from build123d import *

# Parameters (mm, degrees)
SKETCH1_W                                        = 76.2
SKETCH1_H                                        = 50.8
BOSS_EXTRUDE1_DEPTH                              = 11.79269038
BOSS_EXTRUDE2_START                              = -38.1
BOSS_EXTRUDE2_DEPTH                              = 19.05
F_1_4_CLEARANCE_HOLE2_D                          = 6.7564
CBORE_FOR_1_4_SOCKET_HEAD_CAP_SCREW1_D           = 6.7564
CBORE_FOR_1_4_SOCKET_HEAD_CAP_SCREW1_CBORE_D     = 11.1125
CBORE_FOR_1_4_SOCKET_HEAD_CAP_SCREW1_CBORE_DEPTH = 6.35


with BuildPart() as part:
    # Sketch1 → Boss-Extrude1 (new body)
    with BuildSketch(Plane(origin=(0, 0, 0), x_dir=(0, 0, -1), z_dir=(1, 0, 0))):
        Rectangle(SKETCH1_W, SKETCH1_H)
    extrude(amount=BOSS_EXTRUDE1_DEPTH)

    # Sketch7 → Boss-Extrude2 (add, symmetric)
    with BuildSketch(Plane.XY.offset(38.1).offset(BOSS_EXTRUDE2_START)):
        Polygon((11.79269038, -25.4), (49.89269038, -25.4), (49.89269038, 9.525), (43.54269038, 9.525), (43.54269038, -15.875), (11.79269038, -15.875), align=None)
    extrude(amount=BOSS_EXTRUDE2_DEPTH, both=True)

    # 1/4 Clearance Hole2 (through all)
    with Locations(Plane(origin=(49.89269038, 0, 0), x_dir=(0, 0, -1), z_dir=(1, 0, 0))):
        with Locations((-9.525, 3.175), (9.525, 3.175)):
            Hole(F_1_4_CLEARANCE_HOLE2_D / 2)

    # CBORE for 1/4 Socket Head Cap Screw1 (through all)
    with Locations(Plane(origin=(11.79269038, 0, 0), x_dir=(0, 0, -1), z_dir=(1, 0, 0))):
        with Locations((-28.575, 15.875), (28.575, 15.875), (28.575, -15.875), (-28.575, -15.875)):
            CounterBoreHole(CBORE_FOR_1_4_SOCKET_HEAD_CAP_SCREW1_D / 2, CBORE_FOR_1_4_SOCKET_HEAD_CAP_SCREW1_CBORE_D / 2, CBORE_FOR_1_4_SOCKET_HEAD_CAP_SCREW1_CBORE_DEPTH)


solid = part.part
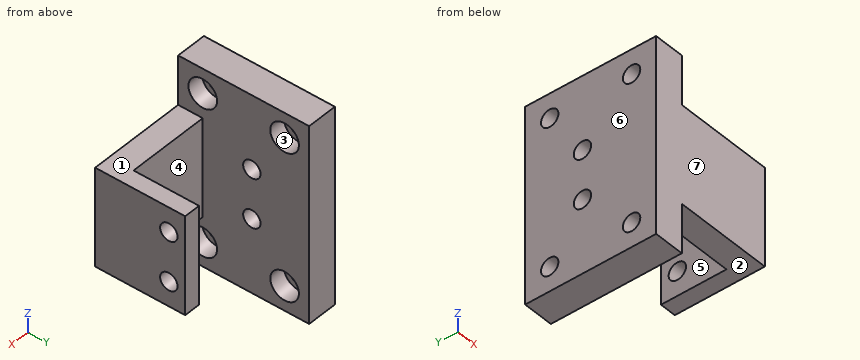
Part model, mm, in its own coordinate system. Face numbers are marked on the shaded views. A direction names the side the tool comes from. Coordinates: 2 decimals unless noted, no trailing zeros. Order: outer loops, then holes, each group sorted by start corner. A loop starts at its lowest first (then second) coordinate and runs counter-clockwise, first axis right, second up. Notation, with made-up numbers: M -9,71 L 12,71 A16 cw 12,99 Z; hole C 59.25,73 d2. An arc over 180 degrees is marked long. One line per question, with ' | ' between items.
Q1. Drill centre lines: line 1 (X direction, y = -9.5, z = -18.5); line 2 (Y direction, x = 24.5, z = -4) (3 decimals); line 3 (Z direction, x = 34.5, y = -21). Where is each one in solid material? Low to high.
A:
line 1: x = 0 to 11.79, 43.54 to 49.89 | line 2: y = -25.4 to -15.875 | line 3: z = -19.05 to 19.05
Q2. 3-axis set-ups, long thin cutter, end or side, ignore diameter. For the marked faces 1, 2, 3 and 4: which of +Z, -Z, +X, -X, +Y, -Y reach the whole face in a straight line?
A:
face 1: +Z, +X, +Y, -Y | face 2: -Z, +X, +Y, -Y | face 3: +X | face 4: +Z, -Z, +Y
Q3. Slice it at A-A (y = -2). Give the cut face in (x, z).
A:
outline: M 0,-38.1 L 11.79,-38.1 L 11.79,38.1 L 0,38.1 Z; M 43.54,-19.05 L 49.89,-19.05 L 49.89,19.05 L 43.54,19.05 Z
Q4. Slice it at D-D (z = -11). Give the cut face in (x, y) (3 decimals).
A:
outline: M 0,-25.4 L 49.893,-25.4 L 49.893,0.136 L 43.543,0.136 L 43.543,-15.875 L 11.793,-15.875 L 11.793,0.136 L 0,0.136 Z; M 0,6.214 L 11.793,6.214 L 11.793,25.4 L 0,25.4 Z; M 43.543,6.214 L 49.893,6.214 L 49.893,9.525 L 43.543,9.525 Z
Q5. Slice it at C-C (y = 17). Give the cut face in (x, z), and give its area (3 significant figures).
A:
outline: M 0,-38.1 L 11.79,-38.1 L 11.79,-34.02 L 5.44,-34.02 L 5.44,-31.76 L 0,-31.76 Z; M 0,-25.39 L 5.44,-25.39 L 5.44,-23.13 L 11.79,-23.13 L 11.79,23.13 L 5.44,23.13 L 5.44,25.39 L 0,25.39 Z; M 0,31.76 L 5.44,31.76 L 5.44,34.02 L 11.79,34.02 L 11.79,38.1 L 0,38.1 Z | area: 691 mm^2
Q6. Two-plate mould, pull along X, no slides. Class the marked faces 5, 6 and 7: +X half, -X half, draft (parallel to the pull), parting line (faces both ways), or undercut.
A:
face 5: undercut | face 6: -X half | face 7: draft
Q7. Pin check, flat tips, straight feed: P1, Ø5.5, axis at y = 13, z = 28, coming from the +X side; P2, Ø7, axis at x = 47, z = -7, coming from the +Y side (3 decimals); P3, Ø16, axis at x = 29.5, z = 5, coming from the +Y side (3 decimals). Stop position of each tip, or through.
A:
P1: stops at x = 11.79 | P2: stops at y = 9.525 | P3: stops at y = -15.875
Q8. Slice it at B-B (z = 2). Give the cut face in (x, y) (3 decimals), and give its area (3 significant figures).
A:
outline: M 0,-25.4 L 49.893,-25.4 L 49.893,9.525 L 43.543,9.525 L 43.543,-15.875 L 11.793,-15.875 L 11.793,25.4 L 0,25.4 Z | area: 1,120 mm^2
